```python
from build123d import *

# Parameters (mm, degrees)
F0_R     = 4
F1_DEPTH = 4
F2_R     = 2.25
F3_DEPTH = 15
F5_DEPTH = 4
F6_R     = 1
F7_R     = 0.5


with BuildPart() as f1:
    # F0 (on Top) → F1 (new body)
    with BuildSketch(Plane.XY):
        Circle(F0_R)
    extrude(amount=F1_DEPTH)

    # F2 (on face) → F3 (join)
    with BuildSketch(Plane(origin=(0, 0, 0), x_dir=(1, 0, 0), z_dir=(0, 0, -1))):
        Circle(F2_R)
    extrude(amount=F3_DEPTH)

    # F4 (on face) → F5 (cut)
    with BuildSketch(Plane.XY.offset(4)):
        Polygon((5.111386, -2.251241), (-4.930368, -2.251241), (-2.237212, -4.44078), (3.483612, -4.44078), align=None)
    extrude(amount=-F5_DEPTH, mode=Mode.SUBTRACT)

    # F6
    f6_edges = [f1.edges().sort_by_distance(p)[0] for p in [
        (-2.25, 0, -15),
    ]]
    fillet(f6_edges, radius=F6_R)

    # F7
    f7_edges = [f1.edges().sort_by_distance(p)[0] for p in [
        (0, 4, 0),
        (0, 4, 4),
    ]]
    fillet(f7_edges, radius=F7_R)


solid = f1.part
```
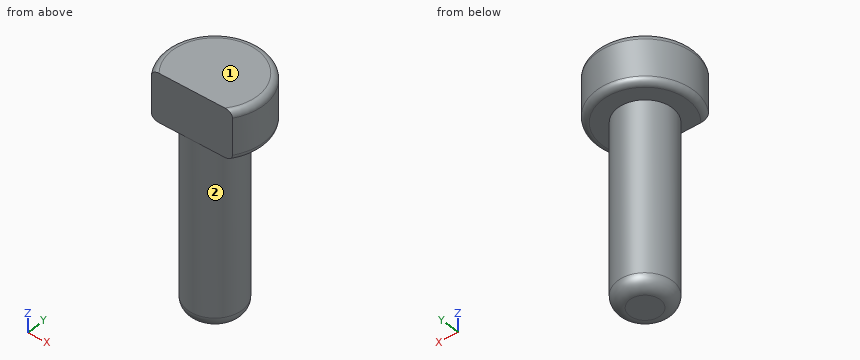
Geometry: final body of the model. Coordinates: model frame, mm. Face numbers are marked on the shaded views. A direction names the side the tool comes from. Coordinates: 2 decimals unless noted, no trailing zeros. Order: outer loops, then holes, each group sorted by start corner. A loop starts at its lowest first (then second) coordinate and runs counter-clockwise, first axis right, second up. Notation, with made-up numbers: (22.25, -24.5) - (63.25, -24.5) arc R22 cw to (63.25, 12.5) - close; hole circle Ø8 at (7.5, 18.25). An arc over 180 degrees is marked (long way). Return JSON: item names as keys, results as strings. Group by question number.
1. Cut plane C-C (z = -9). Output: boundary loops of the cut face in (x, y).
2. Pin query (flat end, axial travel): pin 1 (3 mm diameter, centred on x = -3, y = -0.5, fed in from -Z); pin 2 (1 mm diameter, centred on y = 0.5, z = -4.5, fed in from +X). Return the tip coordinate at first contact, or that it passes through.
3. Material intervals for line 1 along Z through (x, y) = (1.25, 3); line 2 along Y through (x, z) = (0, -9.5); line 3 along Y through (x, z) = (-0.75, -11), sorted ascending. Write a range as [from, to].
4. Cut plane B-B (y = 0). Output: boundary loops of the cut face in (x, z).
5. Set-up query: the marked faces 1 and 2. Return all of +Z, -Z, +X, -X, +Y, -Y with unobstructed straight access to the full face (end or side cutting, diameter ignored); none if empty.
Resolved:
{
 "1": {"outline": "circle Ø4.5 at (0, 0)"},
 "2": {"pin 1": "stops at z = -14.96", "pin 2": "stops at x = 2.25"},
 "3": {"line 1": "z = [0, 4]", "line 2": "y = [-2.25, 2.25]", "line 3": "y = [-2.12, 2.12]"},
 "4": {"outline": "(-4, 0.5) arc R0.5 ccw to (-3.5, 0) - (-2.25, 0) - (-2.25, -14) arc R1 ccw to (-1.25, -15) - (1.25, -15) arc R1 ccw to (2.25, -14) - (2.25, 0) - (3.5, 0) arc R0.5 ccw to (4, 0.5) - (4, 3.5) arc R0.5 ccw to (3.5, 4) - (-3.5, 4) arc R0.5 ccw to (-4, 3.5) - close"},
 "5": {"face 1": "+Z, +X, -X, +Y, -Y", "face 2": "-Z"}
}
